The listing builds one solid part. Answer for the finished solid, in the listing's coordinates (mm). A direction names the side the tool comes from. Give positions to 0.01 mm unless a question says otherwise; leave off trailing zeros. Write each loop counter-clockwise with the first axis right and the second up, starting at its lowest first coordinate (ties: lowest second). Pieces come first, ordered by that corner, then holes. Notation, with made-up numbers: (-38, 74.25) - (-23, 74.25) arc R15 ccw to (-23, 100.25) - close; hole circle Ø4 at (-38, -22). An arc over 180 degrees is marked (long way). Return JSON: item names as keys, results as strings.
from build123d import *

# Parameters (mm, degrees)
SKETCH1_R           = 15.55
BOSS_EXTRUDE1_DEPTH = 1
CHAMFER2_SIZE       = 1
SKETCH4_R           = 3
BOSS_EXTRUDE2_DEPTH = 97.8
FILLET1_R           = 12
SKETCH5_W           = 0.5
SKETCH5_H           = 1


# Some blends are built 0.0001 mm under size
with BuildPart() as part:
    # Sketch1 → Boss-Extrude1 (new body)
    with BuildSketch(Plane(origin=(0, 0, 0), x_dir=(1, 0, 0), z_dir=(0, 1, 0))):
        with Locations(Location((0, 0, 0), (0, 0, 270))):
            Circle(SKETCH1_R)
    extrude(amount=BOSS_EXTRUDE1_DEPTH)

    # Chamfer2
    chamfer2_edges = [part.edges().sort_by_distance(p)[0] for p in [
        (0, 1, -15.55),
    ]]
    chamfer(chamfer2_edges, length=CHAMFER2_SIZE - 0.0001)  # a hair under: the kernel refuses the full size

    # Sketch4 → Boss-Extrude2 (add)
    with BuildSketch(Plane(origin=(0, 1, 0), x_dir=(1, 0, 0), z_dir=(0, 1, 0))):
        with Locations(Location((0, 0, 0), (0, 0, 270))):
            Circle(SKETCH4_R)
    extrude(amount=BOSS_EXTRUDE2_DEPTH)

    # Fillet1
    # the kernel refuses this fillet: 12 mm, written as the material it adds along each edge
    with BuildSketch(Plane(origin=(0, 1, 0), x_dir=(0, 0, 1), z_dir=(-1, 0, 0))) as fillet1_piece_1:
        with BuildLine():
            CenterArc((15, 11.991563284), FILLET1_R, 180, 87.851382174)
            Line((3, 11.991563284), (2.76, 11.991563284))
            Line((2.76, 11.991563284), (2.76, 0))
            Line((2.76, 0), (3, -0.24))
            ThreePointArc((3, -0.24), (8.77505, -0.24), (14.541102, -0.239831266))
            Line((14.541102, -0.239831266), (14.5501, 0))
        make_face()
    revolve(axis=Axis((0, 1, 0), (0, 1, 0)))

    # Sketch5 → Cut-Revolve1 (revolve, cut)
    with BuildSketch(Plane.XY, mode=Mode.PRIVATE) as cut_revolve1_sk:
        with Locations((-2.75, 93.3)):
            Rectangle(SKETCH5_W, SKETCH5_H)
        with Locations((-2.75, 91.3)):
            Rectangle(SKETCH5_W, SKETCH5_H)
        with Locations((-2.75, 89.3)):
            Rectangle(SKETCH5_W, SKETCH5_H)
    revolve(cut_revolve1_sk.sketch.rotate(Axis((0, 98.8, 0), (0, -1, 0)), 270), axis=Axis((0, 98.8, 0), (0, -1, 0)), mode=Mode.SUBTRACT)


solid = part.part
Item 1: Consider L1, parallel to Z at x = -2, y = 52.5; L2, parallel to Y at x = -8, z = 7; L3, parallel to Y at x = -8, z = -13. Determine where each line is inside the solid, lowest interval first.
Answer below:
{"L1": "z = -2.24 to 2.24", "L2": "y = 0 to 1.82", "L3": "y = 0 to 0.29"}
Item 2: Flat-ended cylindrical pins translate along their axes: P1, Ø1.5, axis at y = 51, z = -3.5, coming from the -X side; P2, Ø12, axis at y = 69.5, z = -1, coming from the +X side; P3, Ø1, axis at x = 5, z = 4.5, coming from the +Y side. Find the tip coordinate at first contact, or state that the pin passes through.
Answer below:
{"P1": "stops at x = -1.2", "P2": "stops at x = 3", "P3": "stops at y = 4.8"}
Item 3: The mould has two halves that part along Y. Classify faces 4 (the face through (0, 98.8, 0)), 5 (the face through (0.9, 50.37, 2.86)), 6 (the face through (-2, 93.8, -2)): +Y half, -Y half, draft (parallel to the pull), parting line (faces both ways), or undercut.
Answer below:
{"face 4": "+Y half", "face 5": "draft", "face 6": "undercut"}
Item 4: A cutting plane is placed at C-C on y = 81. Determine the outline of the cut face in (x, z).
Answer below:
{"outline": "circle Ø6 at (0, 0)"}
Item 5: For faces 1 (the face through (2.44, 93.31, -0.54)), 2 (the face through (0.9, 92.29, 2.86)), 3 (the face through (0, 0, 0)), determine the directions among +Z, -Z, +X, -X, +Y, -Y from which every point of the face is accessible in a straight line to the end or side of a thin tool.
Answer below:
{"face 1": "none", "face 2": "+Y", "face 3": "+Z, -Z, +X, -X, -Y"}
